Design review of the part built by this model. Coordinates are the model's own, in mm. Face numbers are marked on the shaded views. A direction names the side the tool comes from. Coordinates: 2 decimals unless noted, no trailing zeros. Order: outer loops, then holes, each group sorted by start corner. A loop starts at its lowest first (then second) coordinate and runs counter-clockwise, first axis right, second up. Notation, with made-up numbers: M 9.5,84.5 L 29.5,84.5 A20 ccw 29.5,106.5 Z; hole C -17.75,21.5 d1. An arc over 180 degrees is marked long. Answer in a Markdown table with one row per item.
from build123d import *

# Parameters (mm, degrees)
SKETCH1_W           = 20
SKETCH1_H           = 6
BOSS_EXTRUDE1_DEPTH = 40
SKETCH5_R           = 6
BOSS_EXTRUDE8_DEPTH = 69
SKETCH8_R           = 8.5
BOSS_EXTRUDE9_DEPTH = 4
FILLET1_R           = 2


with BuildPart() as part:
    # Sketch1 → Boss-Extrude1 (new body)
    with BuildSketch(Plane(origin=(0, 0, 0), x_dir=(1, 0, 0), z_dir=(0, 1, 0))):
        Rectangle(SKETCH1_W, SKETCH1_H)
    extrude(amount=BOSS_EXTRUDE1_DEPTH)

    # Sketch5 → Boss-Extrude8 (add)
    with BuildSketch(Plane.XY.offset(3)):
        with Locations((0, 27.25)):
            Circle(SKETCH5_R)
    extrude(amount=BOSS_EXTRUDE8_DEPTH)

    # Sketch8 → Boss-Extrude9 (add)
    with BuildSketch(Plane.XY.offset(3)):
        with Locations((0, 27.25)):
            Circle(SKETCH8_R)
    extrude(amount=BOSS_EXTRUDE9_DEPTH)

    # Fillet1
    fillet1_edges = [part.edges().sort_by_distance(p)[0] for p in [
        (-10, 20, -3),
        (10, 20, -3),
        (10, 20, 3),
        (-10, 20, 3),
    ]]
    fillet(fillet1_edges, radius=FILLET1_R)


solid = part.part
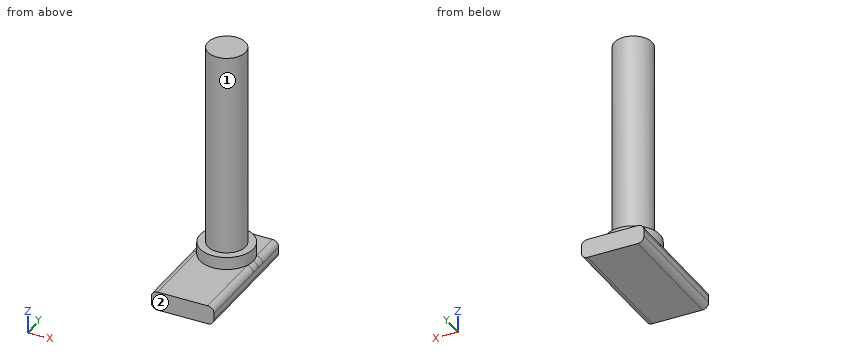
(1) For line 1 along Z through (x, y) = (3.75, 7); line 2 along Y through (x, z) = (0, 50); line 3 along X through (y, z) = (2.5, 2.5), list the stretches that pass through material, from the lowest coordinate up. Write a range as from..to.
Return value:
| item | result |
|---|---|
| line 1 | z = -3..3 |
| line 2 | y = 21.25..33.25 |
| line 3 | x = -9.32..9.32 |
(2) For the marked faces 1 and 2, list the 3-axis set-ups (+Z, -Z, +X, -X, +Y, -Y) from which the entire face can be reached by the end or side of a thin tool; tool diameter is ignored.
Return value:
| item | result |
|---|---|
| face 1 | +Z |
| face 2 | +Z, -Z, +X, -X, -Y |
(3) Add section C-C, the plane z = 61.5. Give the boundary of the cut face in (x, y).
Return value:
| item | result |
|---|---|
| outline | C 0,27.25 d12 |
(4) Add section B-B, the plane x = 0. Give the boundary of the cut face in (y, z).
Return value:
| item | result |
|---|---|
| outline | M 0,-3 L 40,-3 L 40,3 L 35.75,3 L 35.75,7 L 33.25,7 L 33.25,72 L 21.25,72 L 21.25,7 L 18.75,7 L 18.75,3 L 0,3 Z |
(5) Add section D-D, the plane x = -6.75. Give the boundary of the cut face in (y, z), and give its area (3 significant figures).
Return value:
| item | result |
|---|---|
| outline | M 0,-3 L 40,-3 L 40,3 L 32.42,3 L 32.42,7 L 22.08,7 L 22.08,3 L 0,3 Z |
| area | 281 mm2 |
(6) Add section A-A, the plane y = 37.5. Give the boundary of the cut face in (x, z), and give its area (3 significant figures).
Return value:
| item | result |
|---|---|
| outline | M -10,-1 A2 ccw -8,-3 L 8,-3 A2 ccw 10,-1 L 10,1 A2 ccw 8,3 L -8,3 A2 ccw -10,1 Z |
| area | 117 mm2 |
(7) Insertion check: pin 1 Ø10 at (y, z) = (18, 46.5) entering from +X; pin 2 Ø12 at (x, z) = (-3.5, 47) entering from -Y; pin 3 Ø1 at (x, y) = (-6, 34) entering from +Z; pin 4 Ø11 at (x, y) = (-1, 33.5) entering from +Z. Each pin has a flat end and moves straight along its axis. Give the tip position at first contact, or say it passes through.
Return value:
| item | result |
|---|---|
| pin 1 | stops at x = 4.24 |
| pin 2 | stops at y = 21.25 |
| pin 3 | stops at z = 3 |
| pin 4 | stops at z = 72 |
